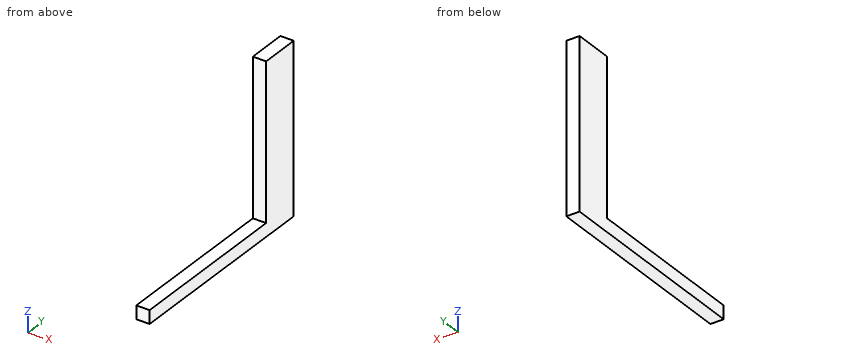
Autodesk Inventor part; units mm, degrees
ref_plane "YZ Plane" through (0, 0, 0) normal (1, 0, 0) x (0, 1, 0)
ref_plane "XZ Plane" through (0, 0, 0) normal (0, 1, 0) x (-1, 0, 0)
ref_plane "XY Plane" through (0, 0, 0) normal (0, 0, 1) x (1, 0, 0)
sketch "Sketch1" plane through (0, 0, 0) normal (0, 0, 1) x (1, 0, 0)
  line L0 (0, 0) -> (7.62, 0)
  line L1 (7.62, 0) -> (7.62, -22.86)
  line L2 (7.62, -22.86) -> (0, -22.86)
  line L3 (0, -22.86) -> (0, 0)
  line L4 (7.62, -22.86) -> (0, -22.86)
  line L5 (0, -22.86) -> (0, -119.38)
  line L6 (0, -119.38) -> (7.62, -119.38)
  line L7 (7.62, -119.38) -> (7.62, -22.86)
  line L8 (0, -111.76) -> (0, -119.38)
  line L9 (0, 0) -> (7.62, 0)
  line L10 (7.62, 0) -> (7.62, -22.86)
  line L11 (7.62, -22.86) -> (0, -22.86)
  line L12 (0, -22.86) -> (0, 0)
  line L13 (7.62, -119.38) -> (35.0744, -119.38)
  line L14 (35.0744, -119.38) -> (69.9139, -119.38)
  line L15 (69.9139, -111.76) -> (69.9139, -119.38)
  line L16 (69.9139, -111.76) -> (7.62, -111.76)
  point P0 (0, -22.86)
  dimension "d0" = 7.62
  dimension "d1" = 22.86
  dimension "d2" = 7.62
  dimension "d3" = 96.52
  dimension "d6" = 7.62
extrude "Extrusion1" add sketch "Sketch1" along normal blind 7.62 contours L0 L1 L2 L3 | L2 L7 L6 L5
extrude "Extrusion2" add sketch "Sketch1" along normal blind 96.52 contours L0 L1 L2 L3
sketch "Sketch2" plane through (0, -119.38, 0) normal (-1, 0, 0) x (0, 0, 1)
  line L0 (0, 0) -> (7.62, 0)
  line L1 (7.62, 0) -> (63.8725, 0)
  line L2 (63.8725, 0) -> (63.8725, 11.8579)
  line L3 (63.8725, 11.8579) -> (7.62, 11.8579)
  point P0 (0, 119.38)
equation "\"d0\" = d6"
properties part number "e"
Check sheet for the modelled part. Datum: model origin and axes. Units: mm. Give positions to 0.01 mm unless a question says otherwise; leave off trailing zeros. Write each loop counter-clockwise with the first axis right and the second up, starting at its lowest first coordinate (ties: lowest second). Pieces come first, ordered by that corner, then holes. Notation, with made-up numbers: (81.25, 83) -> (129.25, 83) arc R7 cw to (129.25, 89) -> close; hole circle Ø8 at (42.5, -28.75). An arc over 180 degrees is marked (long way). Use one line per item in the form item = value. Start each with the question number.
1. Section check A-A (x = 2.75). Record the cut outline in (y, z).
2. Thickness scan on line 1 along Y through (x, z) = (6.75, 56.5); line 2 along Z through (x, y) = (4, -93). Record the ranges inside material, lowest first. Write a range as from..to.
3. Go/stop test with flat-tipped pins: P1, Ø4, axis at x = 2.5, z = 47, coming from the -Y side; P2, Ø3, axis at x = 4.5, y = -93.5, coming from the +Z side; P3, Ø3, axis at x = 5, y = -33.5, coming from the -Z side. Record where each tip stops, or that it passes through.
4. Section check C-C (y = -97.5). Record the cut outline in (x, z), and give its area (3 significant figures).
5. Section check B-B (z = 54.5). Record the cut outline in (x, y), and give its area (3 significant figures).
Conclusion:
q1.outline = (-119.38, 0) -> (0, 0) -> (0, 96.52) -> (-22.86, 96.52) -> (-22.86, 7.62) -> (-119.38, 7.62) -> close
q2.line_1 = -22.86..0
q2.line_2 = 0..7.62
q3.P1 = -22.86
q3.P2 = 7.62
q3.P3 = 0
q4.outline = (0, 0) -> (7.62, 0) -> (7.62, 7.62) -> (0, 7.62) -> close
q4.area = 58.1 mm²
q5.outline = (0, -22.86) -> (7.62, -22.86) -> (7.62, 0) -> (0, 0) -> close
q5.area = 174 mm²
